from build123d import *

# Parameters (mm, degrees)
SKETCH1_W           = 6
SKETCH1_H           = 6
BOSS_EXTRUDE1_DEPTH = 5
CUT_EXTRUDE3_DEPTH  = 13.5
CUT_EXTRUDE4_DEPTH  = 3


with BuildPart() as part:
    # Sketch1 → Boss-Extrude1 (new body)
    with BuildSketch(Plane(origin=(0, 0, 0), x_dir=(1, 0, 0), z_dir=(0, 1, 0))):
        Rectangle(SKETCH1_W, SKETCH1_H)
    extrude(amount=BOSS_EXTRUDE1_DEPTH)

    # Sketch5 → Cut-Extrude3 (cut)
    with BuildSketch(Plane.XY.offset(3)):
        Polygon((-3, 5), (0, 3), (3, 5), align=None)
        Polygon((0, 3), (-3, 5), (-3, 4), align=None)
    extrude(amount=-CUT_EXTRUDE3_DEPTH, mode=Mode.SUBTRACT)

    # Sketch7 → Cut-Extrude4 (cut)
    with BuildSketch(Plane(origin=(0, 0, -3), x_dir=(-1, 0, 0), z_dir=(0, 0, -1))):
        Polygon((0, 3), (3, 0), (3, 6), align=None)
    extrude(amount=-CUT_EXTRUDE4_DEPTH, mode=Mode.SUBTRACT)


solid = part.part
Could you check a few things on this model? Use its own coordinates, in mm. A direction names the side the tool comes from. Round coordinates to 2 decimals unless told otherwise and drop trailing zeros. Write each loop counter-clockwise with the first axis right and the second up, starting at its lowest first coordinate (ties: lowest second). Pieces come first, ordered by that corner, then holes. Notation, with made-up numbers: (11.25, 59.25) - (57.25, 59.25) arc R23 ccw to (57.25, 86.25) - close; hole circle Ø7 at (18, 5). An arc over 180 degrees is marked (long way). Use a Markdown table: item, result.
Q1. For pin 1 (1.5 mm diameter, centred on x = -1.5, z = -1, fed in from +Y); pin 2 (1.5 mm diameter, centred on x = -2, y = 2, fed in from -Z), each with a flat end and sliding along its axis, tell me the tip position at first contact or that it passes through.
Output values:
| item | result |
|---|---|
| pin 1 | y = 2.25 |
| pin 2 | z = -3 |
Q2. I want a section at C-C (x = -1.65). List the corners of the cut face in (y, z) for me.
Output values:
| item | result |
|---|---|
| outline | (0, -3) - (1.35, -3) - (1.35, 0) - (3.55, 0) - (3.55, 3) - (0, 3) - close |
Q3. I want a section at B-B (z = 0.75). List the corners of the cut face in (x, y) for me, plus the area to 3 significant figures.
Output values:
| item | result |
|---|---|
| outline | (-3, 0) - (3, 0) - (3, 5) - (0, 3) - (-3, 4) - close |
| area | 22.5 mm2 |
Q4. Thinking about a two-plate mould opening in X: for faces 4 (the flat face through (-1.5, 3.5, 1.5)), 5 (the flat face through (3, 2, 0)), 6 (the flat face through (0, 0, 0)), which applies, released by +X, released by -X, zero draft, split by the parting line, or undercut?
Output values:
| item | result |
|---|---|
| face 4 | undercut |
| face 5 | released by +X |
| face 6 | zero draft |
Q5. For faces 1 (the flat face through (0, 2, 3)), 2 (the flat face through (-1, 2, -2)), 3 (the flat face through (1.5, 4, 0)), which set-ups out of +Z, -Z, +X, -X, +Y, -Y let a thin tool reach every point of the face, with its end or its side?
Output values:
| item | result |
|---|---|
| face 1 | +Z, +X, -X, +Y, -Y |
| face 2 | -Z, -X, +Y |
| face 3 | +Z, -Z, +Y |
Q6. I want a section at A-A (y = 0.7). List the corners of the cut face in (x, z) for me.
Output values:
| item | result |
|---|---|
| outline | (-3, 0) - (-2.3, 0) - (-2.3, -3) - (3, -3) - (3, 3) - (-3, 3) - close |
Q7. I want a section at D-D (y = 4.4). List the corners of the cut face in (x, z) for me.
Output values:
| item | result |
|---|---|
| outline | (2.1, -3) - (3, -3) - (3, 3) - (2.1, 3) - close |
Q8. Please list where these lines run through material, in increasing order: L1, parallel to Y at x = -0.1, z = -0.7; L2, parallel to Y at x = -0.9, z = 1.7; L3, parallel to X at y = 1.4, z = -1.5.
Output values:
| item | result |
|---|---|
| L1 | 0 to 2.9 |
| L2 | 0 to 3.3 |
| L3 | -1.6 to 3 |
